For this review, take the finished solid that the model builds, in its own axes (mm). A direction names the side the tool comes from. Coordinates: 2 decimals unless noted, no trailing zeros. Write each loop counter-clockwise with the first axis right and the second up, starting at its lowest first coordinate (ties: lowest second). Pieces come first, ordered by that corner, then holes. Notation, with made-up numbers: (-14.75, 51.5) - (14.25, 51.5) arc R7 ccw to (14.25, 60.5) - close; hole circle Ø2 at (77.25, 4). An arc over 180 degrees is marked (long way). Write each question's results on one line, items separated by ' | '.
Autodesk Inventor part; units mm, degrees
ref_plane "YZ Plane" through (0, 0, 0) normal (1, 0, 0) x (0, 1, 0)
ref_plane "XZ Plane" through (0, 0, 0) normal (0, 1, 0) x (-1, 0, 0)
ref_plane "XY Plane" through (0, 0, 0) normal (0, 0, 1) x (1, 0, 0)
sketch "草圖1" plane through (0, 0, 0) normal (1, 0, 0) x (0, 1, 0)
  line L0 (2, 1.1547) -> (2, 10)
  line L1 (2, 10) -> (4, 10)
  line L2 (4, 10) -> (4, 13)
  line L3 (3, 15) -> (6, 20)
  line L4 (6, 20) -> (7.5, 20)
  arc A0 (7.3358, 14.0988) -> (7.3358, 14.0988) centre (-51.8892, 10.8387) ccw
  line L5 (7.5, 20) -> (7.5, 0)
  line L6 (0, -10) -> (0, 12.2342)
  line L7 (4, 13) -> (3, 13)
  line L8 (3, 13) -> (3, 15)
  line L9 (2, 1.1547) -> (0, 0)
  line L10 (0, 0) -> (7.5, 0)
  dimension "d3" = 8
  dimension "d4" = 4
  dimension "d5" = 15
  dimension "d6" = 12
  dimension "d7" = 6
  dimension "d8" = 5
  dimension "d9" = 7
  dimension "d10" = 3
  dimension "d11" = 0
  dimension "d19" = 20
  dimension "d24" = 20
  dimension "d25" = 0
  dimension "d27" = 60
revolve "迴轉1" add sketch "草圖1" angle 180 about axis through (0, 0, -10) along (0, 0, 1) picked at (3.6603, 4.915) contours L0 L1 L2 L7 L8 L3 L4 A0 L10 L9 | A0 L4 L5 L10
sketch "草圖3" plane through (0, 0, 0) normal (0, 0, -1) x (-1, 0, 0)
  line L0 (0, -7.5) -> (0, 0)
  arc A0 (0, -7.5) -> (0, 7.5) centre (0, 0) ccw
  line L1 (-11.5773, 0) -> (12.4556, 0) construction
  line L2 (0.0279, 7.6444) -> (0.0279, -10.5735) construction
  line L3 (5.7735, 10) -> (11.547, 0)
  line L4 (11.547, 0) -> (5.7735, -10)
  line L5 (5.7735, -10) -> (0.0248, -10)
  line L6 (0, 10) -> (5.7735, 10)
  line L7 (-0.0017, 11.3448) -> (0.0279, -12.4793) construction
  line L8 (0.0248, -10) -> (0, 10)
  point P0 (6.4952, 3.75)
  dimension "d29" = 20
  dimension "d32" = 2.5
extrude "擠出1" add sketch "草圖3" along normal blind 10
properties part number "示範一"
Q1. Wall thickness on line 1 along Z through (x, y) = (-11, 0); line 2 along Y through (x, z) = (-0.25, 16); line 3 along Y through (x, z) = (-0.5, 3.5): over which ranges is each line inside the solid? List them lowest first. Write a range as from..to.
Results found:
line 1: -10..0 | line 2: -7.5..-3.59, 3.59..7.5 | line 3: -7.48..-1.94, 1.94..7.48
Q2. Mouldability with a two-part tool opening along Z and no side actions: class faces 5 (the face through (-3.4, -0.1, 13)), 6 (the face through (-4, 0, 12)), 7 (the face through (-3, 10, -5)), 8 (the face through (-8, 0, 0)) as pulls with the +Z half, pulls with the -Z half, needs draft (parallel to the pull), parting line crosses it, or undercut.
Results found:
face 5: undercut | face 6: undercut | face 7: needs draft | face 8: pulls with the +Z half
Q3. For faces 1 (the face through (-2.5, -0.1, 10)), 2 (the face through (-7.5, -0.16, 9.86)), 3 (the face through (-2, 0, 6)), 4 (the face through (-8.62, 5.07, -4.93)), list the 3-axis set-ups (+Z, -Z, +X, -X, +Y, -Y) from which the entire face can be reached by the end or side of a thin tool; tool diameter is ignored.
Results found:
face 1: +X | face 2: +Z, -X | face 3: +Z, +X | face 4: +Z, -Z, -X, +Y
Q4. Take a section at B-B on y = 9.25. State the section outline as (x, z) points, plus the area to 3 significant figures.
Results found:
outline: (-6.21, -10) - (0, -10) - (0, 0) - (-6.21, 0) - close | area: 62.1 mm2
Q5. Take a section at A-A on z = 10.5. State the section outline as (x, y) points, plus the area to 3 significant figures.
Results found:
outline: (0, -7.5) - (0, -4) arc R4 cw to (0, 4) - (0, 7.5) arc R7.5 ccw to start | area: 63.2 mm2
Q6. For pin 1 (4.5 mm diameter, centred on x = -2, y = 2, fed in from +Z); pin 2 (3 mm diameter, centred on x = -4.5, z = 6.5, fed in from +Y); pin 3 (2 mm diameter, centred on x = -8, y = -6.5, fed in from +Z), all flat-tipped, find the tip position at first contact; note any pin that passes through.
Results found:
pin 1: z = 18.46 | pin 2: y = 6.87 | pin 3: z = 0
